The listing builds one solid part. Answer for the finished solid, in the listing's coordinates (mm). Face numbers are marked on the shaded views. Give positions to 0.01 mm unless a question says otherwise; leave off trailing zeros. Loops run counter-clockwise (first coordinate to the right, second up) from the corner with the lowest first, then second, coordinate; pieces in that order, holes last.
Item 1: Section C-C, the plane z = 0.55 is taken. Give the vertices of the cut face in (x, y), and give its area (3 significant figures).
Item 2: Each of these flat-tipped pins is pushed along its axis until it touches: pin 1 Ø2 at (x, y) = (-22, 0) entering from -Z; pin 2 Ø1 at (x, y) = (20.5, 10.5) entering from -Z; pin 3 Ø1 at (x, z) = (-25.5, 1.5) entering from -Y. Where does it stop, or does it pass through?
Item 3: Section A-A, the plane x = 0 is taken. Give the vertices of the cut face in (y, z) (3 decimals).
Item 4: Section B-B, the plane y = 0 is taken. Give the vertices of the cut face in (x, z) (3 decimals).
Item 5: Section D-D, the plane x = -22 is taken. Give the vertices of the cut face in (y, z) (3 decimals), and give its area (3 significant figures).
Item 6: The mould has two halves that part along Z. Classify the marked faces 1 and 2: pulls with the +Z half, pulls with the -Z half, needs draft (parallel to the pull), parting line crosses it, or undercut.
Item 7: Consider line 1 along Y through (x, z) = (0, 1.1); line 2 along Y through (x, z) = (22, 1.25); line 3 along X through (y, z) = (-23, 1.3). Determine where each line is inside the solid, lowest interval first.
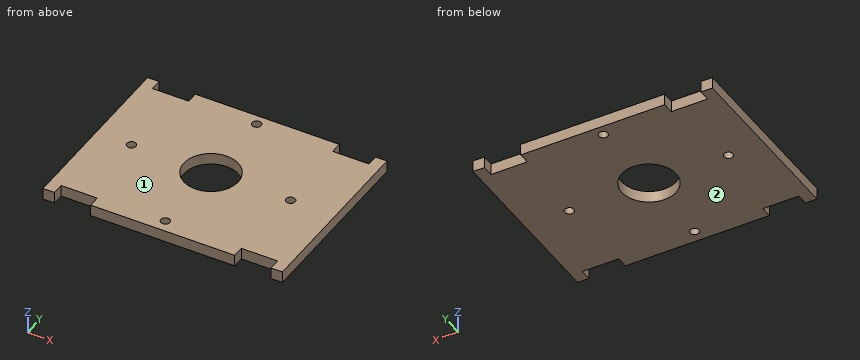
from build123d import *

# Parameters (mm, degrees)
F0_R     = 1.25
F0_R_2   = 7.5
F1_DEPTH = 3.175


with BuildPart() as f1:
    # F0 (on Top) → F1 (new body)
    with BuildSketch(Plane.XY):
        Polygon((-28.653005, 24.935823), (-31.82862, 24.935823), (-31.82862, -25.495171), (-28.653005, -25.495171), (-28.653005, -22.319556), (-18.653005, -22.319556), (-18.653005, -25.495171), (21.170266, -25.495171), (21.170266, -22.319556), (31.170266, -22.319556), (31.170266, -25.495171), (34.34638, -25.495171), (34.34638, 24.935823), (31.170266, 24.935823), (31.170266, 21.760208), (21.170266, 21.760208), (21.170266, 24.935823), (-18.653005, 24.935823), (-18.653005, 21.760208), (-28.653005, 21.760208), align=None)
        with Locations((0, -22)):
            Circle(F0_R, mode=Mode.SUBTRACT)
        with Locations((-22, 0)):
            Circle(F0_R, mode=Mode.SUBTRACT)
        Circle(F0_R_2, mode=Mode.SUBTRACT)
        with Locations((0, 22)):
            Circle(F0_R, mode=Mode.SUBTRACT)
        with Locations((22, 0)):
            Circle(F0_R, mode=Mode.SUBTRACT)
    extrude(amount=F1_DEPTH)


solid = f1.part
Worked answers:
1. outline: (-31.83, -25.5) - (-28.65, -25.5) - (-28.65, -22.32) - (-18.65, -22.32) - (-18.65, -25.5) - (21.17, -25.5) - (21.17, -22.32) - (31.17, -22.32) - (31.17, -25.5) - (34.35, -25.5) - (34.35, 24.94) - (31.17, 24.94) - (31.17, 21.76) - (21.17, 21.76) - (21.17, 24.94) - (-18.65, 24.94) - (-18.65, 21.76) - (-28.65, 21.76) - (-28.65, 24.94) - (-31.83, 24.94) - close; hole circle Ø2.5 at (-22, 0); hole circle Ø15 at (0, 0); hole circle Ø2.5 at (0, -22); hole circle Ø2.5 at (0, 22); hole circle Ø2.5 at (22, 0)
1. area: 3,010 mm2
2. pin 1: passes through
2. pin 2: stops at z = 0
2. pin 3: stops at y = -22.32
3. outline: (-25.495, 0) - (-23.25, 0) - (-23.25, 3.175) - (-25.495, 3.175) - close; (-20.75, 0) - (-7.5, 0) - (-7.5, 3.175) - (-20.75, 3.175) - close; (7.5, 0) - (20.75, 0) - (20.75, 3.175) - (7.5, 3.175) - close; (23.25, 0) - (24.936, 0) - (24.936, 3.175) - (23.25, 3.175) - close
4. outline: (-31.829, 0) - (-23.25, 0) - (-23.25, 3.175) - (-31.829, 3.175) - close; (-20.75, 0) - (-7.5, 0) - (-7.5, 3.175) - (-20.75, 3.175) - close; (7.5, 0) - (20.75, 0) - (20.75, 3.175) - (7.5, 3.175) - close; (23.25, 0) - (34.346, 0) - (34.346, 3.175) - (23.25, 3.175) - close
5. outline: (-22.32, 0) - (-1.25, 0) - (-1.25, 3.175) - (-22.32, 3.175) - close; (1.25, 0) - (21.76, 0) - (21.76, 3.175) - (1.25, 3.175) - close
5. area: 132 mm2
6. face 1: pulls with the +Z half
6. face 2: pulls with the -Z half
7. line 1: y = -25.5 to -23.25, -20.75 to -7.5, 7.5 to 20.75, 23.25 to 24.94
7. line 2: y = -22.32 to -1.25, 1.25 to 21.76
7. line 3: x = -31.83 to -28.65, -18.65 to -0.75, 0.75 to 21.17, 31.17 to 34.35
